Part print with two shaded views. Sizes in mm from the minimum x, y, z corner. A direction names the side the tool comes from. Give positions to 0.01 mm unless a question says otherwise; leave off trailing zeros. Write each loop counter-clockwise with the first axis right and the second up, starting at its lowest first coordinate (ties: lowest second). Pieces come first, ordered by that corner, then holes.
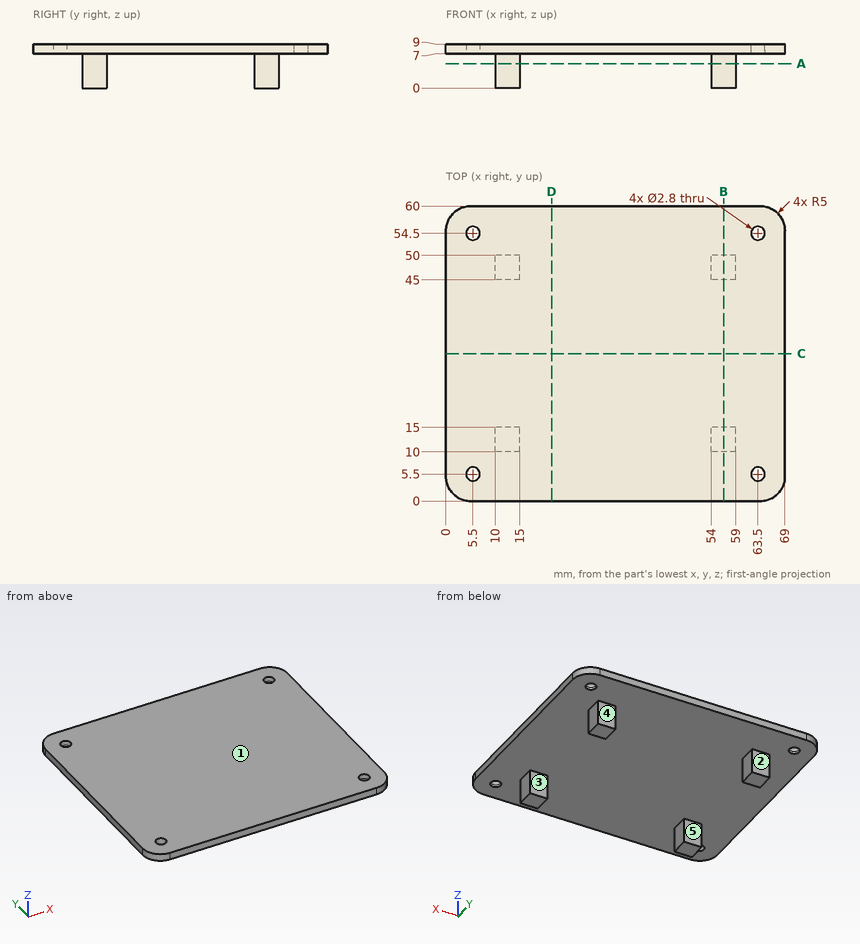
1) Saw through at D-D (x = 21.5). Write the cut outline in (y, z), and give its area (3 significant figures).
Check result:
outline: (0, 7) - (60, 7) - (60, 9) - (0, 9) - close
area: 120 mm2
2) Saw through at B-B (x = 56.5). Write the cut outline in (y, z), and give its area (3 significant figures).
Check result:
outline: (0, 7) - (10, 7) - (10, 0) - (15, 0) - (15, 7) - (45, 7) - (45, 0) - (50, 0) - (50, 7) - (60, 7) - (60, 9) - (0, 9) - close
area: 190 mm2
3) Saw through at A-A (z = 5). Write the cut outline in (x, y).
Check result:
outline: (10, 10) - (15, 10) - (15, 15) - (10, 15) - close; (10, 45) - (15, 45) - (15, 50) - (10, 50) - close; (54, 10) - (59, 10) - (59, 15) - (54, 15) - close; (54, 45) - (59, 45) - (59, 50) - (54, 50) - close
4) Saw through at C-C (y = 30). Write the cut outline in (x, z).
Check result:
outline: (0, 7) - (69, 7) - (69, 9) - (0, 9) - close
5) Drill centre lines: L1, parallel to X at y = 5.5, z = 7.2; L2, parallel to Y at x = 5.5, z = 8.4; L3, parallel to Z at x = 63.5, y = 9. Where is each one in solid material? Low to high.
Check result:
L1: x = 0 to 4.1, 6.9 to 62.1, 64.9 to 69
L2: y = 0 to 4.1, 6.9 to 53.1, 55.9 to 60
L3: z = 7 to 9
6) 3-axis set-ups, long thin cutter, end or side, ignore diameter. For the marked faces 4 and 5: which of +Z, -Z, +X, -X, +Y, -Y reach the whole face in a straight line?
Check result:
face 4: -Z, +X, -X, +Y
face 5: -Z, +X, -X
7) Flat gauge pins, fed straight in: P1, Ø2.5, axis at x = 13, z = 4.5, coming from the -Y side; P2, Ø3, axis at x = 5.5, y = 54.5, coming from the -Z side; P3, Ø1.5, axis at y = 12.5, z = 2, coming from the -X side. Where does each tip first touch, or does it go through?
Check result:
P1: stops at y = 10
P2: stops at z = 7
P3: stops at x = 10
8) Mould opens along Y. For the marked faces 1, 2 and 3 say: +Y half, -Y half, draft (parallel to the pull), parting line (faces both ways), or undercut.
Check result:
face 1: draft
face 2: +Y half
face 3: undercut
